Work out the finished part from the listing and answer in its coordinate system (mm). Face numbers are marked on the shaded views. A direction names the side the tool comes from. Round coordinates to 2 decimals unless told otherwise and drop trailing zeros. Order: outer loops, then holes, each group sorted by start corner. A loop starts at its lowest first (then second) coordinate and runs counter-clockwise, first axis right, second up. Notation, with made-up numbers: (54.5, -25) - (58.5, -25) arc R26 cw to (58.5, 2) - close; hole circle Ø6 at (32, -20). An arc over 180 degrees is marked (long way). Use CSV: the item, a comma, the result in double quotes.
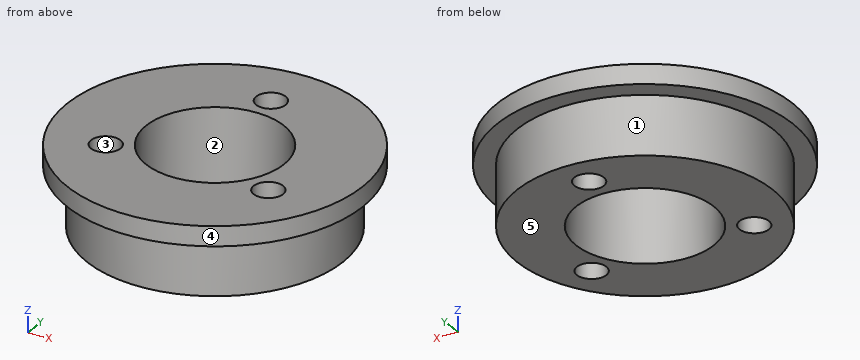
from build123d import *

# Parameters (mm, degrees)
SKETCH1_R           = 13
SKETCH1_R_2         = 7
BOSS_EXTRUDE1_DEPTH = 6
SKETCH2_R           = 15
SKETCH2_R_2         = 7
BOSS_EXTRUDE2_DEPTH = 2
SKETCH3_R           = 1.5
CUT_EXTRUDE1_DEPTH  = 16


with BuildPart() as part:
    # Sketch1 → Boss-Extrude1 (new body)
    with BuildSketch(Plane.XY):
        Circle(SKETCH1_R)
        Circle(SKETCH1_R_2, mode=Mode.SUBTRACT)
    extrude(amount=BOSS_EXTRUDE1_DEPTH)

    # Sketch2 → Boss-Extrude2 (add)
    with BuildSketch(Plane.XY.offset(6)):
        Circle(SKETCH2_R)
        Circle(SKETCH2_R_2, mode=Mode.SUBTRACT)
    extrude(amount=BOSS_EXTRUDE2_DEPTH)

    # Sketch3 → Cut-Extrude1 (cut)
    with BuildSketch(Plane.XY.offset(8)):
        with Locations((0, 9.525)):
            Circle(SKETCH3_R)
        with Locations((8.248891971, -4.7625)):
            Circle(SKETCH3_R)
        with Locations((-8.248891971, -4.7625)):
            Circle(SKETCH3_R)
    extrude(amount=-CUT_EXTRUDE1_DEPTH, mode=Mode.SUBTRACT)


solid = part.part
(1) The mould has two halves that part along X. Classify the marked faces 3, 4 and 5: released by +X, released by -X, zero draft, split by the parting line, or undercut.
Findings below:
face 3,"undercut"
face 4,"split by the parting line"
face 5,"zero draft"
(2) Find section A-A (y = 0). Determine the outline of the cut face in (x, z), and give its area (3 significant figures).
Findings below:
outline,"(-15, 6) - (-13, 6) - (-13, 0) - (-7, 0) - (-7, 8) - (-15, 8) - close; (7, 0) - (13, 0) - (13, 6) - (15, 6) - (15, 8) - (7, 8) - close"
area,"104 mm²"
(3) Find section B-B (x = 0). Determine the outline of the cut face in (y, z) (3 decimals), and give its area (3 significant figures).
Findings below:
outline,"(-15, 6) - (-13, 6) - (-13, 0) - (-7, 0) - (-7, 8) - (-15, 8) - close; (7, 0) - (8.025, 0) - (8.025, 8) - (7, 8) - close; (11.025, 0) - (13, 0) - (13, 6) - (15, 6) - (15, 8) - (11.025, 8) - close"
area,"80.0 mm²"
(4) Find the intervals of material crossed by L1, parallel to Y at x = 0, z = 3.5 (3 decimals); L2, parallel to X at y = -3.5, z = 3.5; L3, parallel to X at y = -0.25, z = 3.5, in increasing order. Write a range as from..to.
Findings below:
L1,"y = -13..-7, 7..8.025, 11.025..13"
L2,"x = -12.52..-9.06, -7.44..-6.06, 6.06..7.44, 9.06..12.52"
L3,"x = -13..-7, 7..13"
(5) For the marked faces 1 and 2, determine the directions among +Z, -Z, +X, -X, +Y, -Y from which every point of the face is accessible in a straight line to the end or side of a thin tool.
Findings below:
face 1,"-Z"
face 2,"+Z, -Z"
(6) This flat-tipped pin is pushed along its axis until it touches: pin 1 (1.5 mm diameter, centred on x = -11.5, z = 7, fed in from -Y). Where does it stop, or does it pass through?
Findings below:
pin 1,"stops at y = -10.46"
(7) Find section C-C (x = -6). Determine the outline of the cut face in (y, z).
Findings below:
outline,"(-13.75, 6) - (-11.53, 6) - (-11.53, 0) - (-3.61, 0) - (-3.61, 8) - (-13.75, 8) - close; (3.61, 0) - (11.53, 0) - (11.53, 6) - (13.75, 6) - (13.75, 8) - (3.61, 8) - close"
(8) Find section D-D (y = 12). Determine the outline of the cut face in (x, z).
Findings below:
outline,"(-9, 6) - (-5, 6) - (-5, 0) - (5, 0) - (5, 6) - (9, 6) - (9, 8) - (-9, 8) - close"
